CAD build for the part. Positions are in the model's coordinates, mm. A direction names the side the tool comes from. Round coordinates to 2 decimals unless told otherwise and drop trailing zeros. Order: outer loops, then holes, each group sorted by start corner. A loop starts at its lowest first (then second) coordinate and runs counter-clockwise, first axis right, second up. Notation, with made-up numbers: M 31.5,-38 L 41.5,-38 A24 cw 41.5,-27 Z; hole C -14,75.25 d7. An arc over 180 degrees is marked long. Answer as a JSON object with one key per item and string values.
```python
from build123d import *

# Parameters (mm, degrees)
BOSS_EXTRU_1_DEPTH                  = 4.8
ENL_V_MAT_EXTRU_1_DEPTH             = 2.3
D_POUILLE1_ANGLE                    = -36.151625355
DIAM_TRE_DU_PER_AGE_3_1_3_1_1_D     = 3.1
DIAM_TRE_DU_PER_AGE_3_1_3_1_1_DEPTH = 4.8
CONG_1_R                            = 10
ESQUISSE5_R                         = 1.55
BOSS_EXTRU_2_DEPTH                  = 4.8
ENL_V_MAT_EXTRU_2_DEPTH             = 78.657948853
ESQUISSE6_W                         = 3
ESQUISSE6_H                         = 3.1
ESQUISSE6_H_2                       = 1.22
ESQUISSE6_W_2                       = 5
ESQUISSE6_H_3                       = 1.23
ENL_V_MAT_EXTRU_3_DEPTH             = 76.557273061
ESQUISSE7_W                         = 5
ESQUISSE7_H                         = 5.8
BOSS_EXTRU_3_DEPTH                  = 4.8
CONG_2_R                            = 3
CONG_3_R                            = 0.5
CHANFREIN1_SIZE                     = 2


with BuildPart() as part:
    # Esquisse1 → Boss.-Extru.1 (new body)
    with BuildSketch(Plane(origin=(0, 0, 0), x_dir=(-1, 0, 0), z_dir=(0, 0, -1))):
        with BuildLine():
            Line((38, -9.9), (38, 60))
            Line((38, 60), (-12, 60))
            Line((-12, 60), (-12, 11.9))
            ThreePointArc((-12, 11.9), (-11, 10.9), (-12, 9.9))
            Line((-12, 9.9), (-17, 9.9))
            Line((-17, 9.9), (-17, 4.1))
            Line((-17, 4.1), (-12, 4.1))
            ThreePointArc((-12, 4.1), (-11, 3.1), (-12, 2.1))
            Line((-12, 2.1), (-12, -2.1))
            ThreePointArc((-12, -2.1), (-11, -3.1), (-12, -4.1))
            Line((-12, -4.1), (-17, -4.1))
            Line((-17, -4.1), (-17, -9.9))
            Line((-17, -9.9), (38, -9.9))
        make_face()
    extrude(amount=-BOSS_EXTRU_1_DEPTH)

    # Esquisse2 → Enl_v. mat.-Extru.1 (cut)
    with BuildSketch(Plane.XY.offset(4.8)):
        with BuildLine():
            Line((-38, -5.25), (7, -5.25))
            ThreePointArc((7, -5.25), (8, -4.25), (7, -3.25))
            Line((7, -3.25), (7, 3.25))
            ThreePointArc((7, 3.25), (8, 4.25), (7, 5.25))
            Line((7, 5.25), (-38, 5.25))
            Line((-38, 5.25), (-38, -5.25))
        make_face()
    extrude(amount=-ENL_V_MAT_EXTRU_1_DEPTH, mode=Mode.SUBTRACT)

    # D_pouille1
    d_pouille1_faces = [part.faces().sort_by_distance(p)[0] for p in [
        (-38, 26.992889488, 2.303049427),
    ]]
    draft(d_pouille1_faces, Plane(origin=(7, 5.25, 2.5), x_dir=(-1, 0, 0), z_dir=(0, -1, 0)), D_POUILLE1_ANGLE)

    # Diam_tre du per_age _3.1 _3.1_1
    with Locations(Plane(origin=(0, 0, 0), x_dir=(-1, 0, 0), z_dir=(0, 0, -1))):
        with Locations((16.5, 0), (31.5, 0)):
            Hole(DIAM_TRE_DU_PER_AGE_3_1_3_1_1_D / 2, depth=DIAM_TRE_DU_PER_AGE_3_1_3_1_1_DEPTH)

    # Cong_1
    cong_1_edges = [part.edges().sort_by_distance(p)[0] for p in [
        (2, 60, 2.4),
    ]]
    fillet(cong_1_edges, radius=CONG_1_R)

    # Esquisse5 → Boss.-Extru.2 (add)
    with BuildSketch(Plane.XY.offset(4.8)):
        with BuildLine():
            Line((-38, 5.25), (-45.671232877, -5.25))
            Line((-45.671232877, -5.25), (7, -5.25))
            ThreePointArc((7, -5.25), (8, -4.25), (7, -3.25))
            Line((7, -3.25), (7, 3.25))
            ThreePointArc((7, 3.25), (8, 4.25), (7, 5.25))
            Line((7, 5.25), (-38, 5.25))
        make_face()
        with Locations(Location((-31.5, 0, 0), (0, 0, 180))):
            Circle(ESQUISSE5_R, mode=Mode.SUBTRACT)
        with Locations(Location((-16.5, 0, 0), (0, 0, 180))):
            Circle(ESQUISSE5_R, mode=Mode.SUBTRACT)
        with BuildLine():
            ThreePointArc((12, -2.1), (11, -3.1), (12, -4.1))
            Line((12, -4.1), (12, -2.1))
        make_face()
        with BuildLine():
            ThreePointArc((12, 4.1), (11, 3.1), (12, 2.1))
            Line((12, 2.1), (12, 4.1))
        make_face()
        with BuildLine():
            Line((12, 9.9), (12, 11.9))
            ThreePointArc((12, 11.9), (11, 10.9), (12, 9.9))
        make_face()
    extrude(amount=-BOSS_EXTRU_2_DEPTH)

    # Esquisse5_4 → Enl_v. mat.-Extru.2 (cut, through all)
    with BuildSketch(Plane.XY.offset(4.8)):
        Polygon((-45.671232877, -9.9), (-45.671232877, -5.25), (-49.068493151, -9.9), align=None)
    extrude(amount=-ENL_V_MAT_EXTRU_2_DEPTH, mode=Mode.SUBTRACT)

    # Esquisse6 → Enl_v. mat.-Extru.3 (cut, through all)
    with BuildSketch(Plane.XY.offset(4.8)):
        with Locations((2.5, 0)):
            Rectangle(ESQUISSE6_W, ESQUISSE6_H)
        with Locations((5.5, 0)):
            Rectangle(ESQUISSE6_W, ESQUISSE6_H)
        with Locations((5.5, -2.16)):
            Rectangle(ESQUISSE6_W, ESQUISSE6_H_2)
        with Locations((9.5, 0)):
            Rectangle(ESQUISSE6_W_2, ESQUISSE6_H)
        with Locations((5.5, 2.165)):
            Rectangle(ESQUISSE6_W, ESQUISSE6_H_3)
        with Locations((5.5, 47.94)):
            Rectangle(ESQUISSE6_W, ESQUISSE6_H_2)
        with Locations((5.5, 50.1)):
            Rectangle(ESQUISSE6_W, ESQUISSE6_H)
        with Locations((2.5, 50.1)):
            Rectangle(ESQUISSE6_W, ESQUISSE6_H)
        with Locations((5.5, 52.265)):
            Rectangle(ESQUISSE6_W, ESQUISSE6_H_3)
        with Locations((9.5, 50.1)):
            Rectangle(ESQUISSE6_W_2, ESQUISSE6_H)
    extrude(amount=-ENL_V_MAT_EXTRU_3_DEPTH, mode=Mode.SUBTRACT)

    # Esquisse7 → Boss.-Extru.3 (add)
    with BuildSketch(Plane.XY.offset(4.8)):
        with Locations((14.5, 57.1)):
            Rectangle(ESQUISSE7_W, ESQUISSE7_H)
        with Locations((14.5, 43.1)):
            Rectangle(ESQUISSE7_W, ESQUISSE7_H)
    extrude(amount=-BOSS_EXTRU_3_DEPTH)

    # Cong_2
    cong_2_edges = [part.edges().sort_by_distance(p)[0] for p in [
        (-45.671232877, -5.25, 2.4),
        (-45.671232877, -9.9, 2.4),
    ]]
    fillet(cong_2_edges, radius=CONG_2_R)

    # Cong_3
    cong_3_edges = [part.edges().sort_by_distance(p)[0] for p in [
        (17, -9.9, 2.4),
        (17, -4.1, 2.4),
        (17, 4.1, 2.4),
        (17, 9.9, 2.4),
        (17, 46, 2.4),
        (17, 40.2, 2.4),
        (17, 60, 2.4),
        (17, 54.2, 2.4),
    ]]
    fillet(cong_3_edges, radius=CONG_3_R)

    # Chanfrein1
    chanfrein1_edges = [part.edges().sort_by_distance(p)[0] for p in [
        (-31.5, 1.55, 0),
        (-16.5, 1.55, 0),
    ]]
    chamfer(chanfrein1_edges, length=CHANFREIN1_SIZE)


solid = part.part
```
Item 1: Two-plate mould, pull along Y, no slides. Class faces 1 (the flat face through (-13, -9.9, 2)), 2 (the flat face through (-8, 18, 0)), 3 (the flat face through (14, 4.1, 2)), 4 (the flat face through (9, -1.55, 2)): released by +Y, released by -Y, zero draft, split by the parting line, or undercut.
Worked answers:
{"face 1": "released by -Y", "face 2": "zero draft", "face 3": "undercut", "face 4": "undercut"}
Item 2: Saw through at B-B on x = -31.5. List the corners of the cut face in (y, z), and give its area (3 significant figures).
Worked answers:
{"outline": "M -9.9,0 L -3.55,0 L -1.55,2 L -1.55,4.8 L -9.9,4.8 Z; M 1.55,2 L 3.55,0 L 14.15,0 L 14.15,4.8 L 1.55,4.8 Z", "area": "96.5 mm2"}
Item 3: Saw through at D-D on x = -24.5. List the corners of the cut face in (y, z).
Worked answers:
{"outline": "M -9.9,0 L 23.73,0 L 23.73,4.8 L -9.9,4.8 Z"}
Item 4: Drop flat-ended pins along their axis: pin 1 Ø1.5 at (x, z) = (2.5, 2.5) entering from +Y; pin 2 Ø1.6 at (y, z) = (49.5, 2.5) entering from +X; pin 3 Ø2.5 at (y, z) = (-0.5, 2.5) entering from +X. Give the stop position or say it passes through.
Worked answers:
{"pin 1": "stops at y = 59.24", "pin 2": "stops at x = 1", "pin 3": "stops at x = 12"}
Item 5: Wall check: line 1 along Y through (x, z) = (7.5, 2.1); line 2 along X through (y, z) = (0, 3.4); line 3 along Y through (x, z) = (6, 3.75). Give the ranges that are in metal, low to high. Write a range as [from, to].
Worked answers:
{"line 1": "y = [-9.9, -1.55], [1.55, 48.55], [51.65, 60]", "line 2": "x = [-41.84, -33.05], [-29.95, -18.05], [-14.95, 1]", "line 3": "y = [-9.9, -2.77], [2.78, 47.33], [52.88, 59.94]"}
Item 6: 3-axis set-ups, long thin cutter, end or side, ignore diameter. For faces 5 (the flat face through (9, 51.65, 2)), 6 (the flat face through (12, 60, 2)): which of +Z, -Z, +X, -X, +Y, -Y reach the whole face in a straight line?
Worked answers:
{"face 5": "+Z, -Z, +X", "face 6": "+Z, -Z, +X, -X, +Y"}
Item 7: Saw through at C-C on y = 28.5. List the corners of the cut face in (x, z).
Worked answers:
{"outline": "M -21.01,0 L 12,0 L 12,4.8 L -21.01,4.8 Z"}
Item 8: Saw through at A-A on x = -16.5. List the corners of the cut face in (y, z).
Worked answers:
{"outline": "M -9.9,0 L -3.55,0 L -1.55,2 L -1.55,4.8 L -9.9,4.8 Z; M 1.55,2 L 3.55,0 L 34.68,0 L 34.68,4.8 L 1.55,4.8 Z"}
